from build123d import *

# Parameters (mm, degrees)
F0_W      = 70
F0_H      = 40
F1_DEPTH  = 40
F3_DEPTH  = 70
F4_DEPTH  = 140
F6_DEPTH  = 40
F8_DEPTH  = 40
F9_DEPTH  = 80
F11_DEPTH = 10


with BuildPart() as f1:
    # F0 (on Front) → F1 (new body)
    with BuildSketch(Plane.XZ):
        with Locations((35, 20)):
            Rectangle(F0_W, F0_H)
    extrude(amount=F1_DEPTH)

    # F2 (on face) → F3 (join)
    with BuildSketch(Plane.YZ.offset(70)):
        Polygon((-20, 40), (-40, 40), (-40, 20), align=None)
    extrude(amount=F3_DEPTH)

    # F3_face (on face) → F4 (cut)
    with BuildSketch(Plane(origin=(140, -33.333333, 33.333333), x_dir=(0, 1, 0), z_dir=(1, 0, 0))):
        Polygon((13.333333, 6.666667), (-6.666667, 6.666667), (-6.666667, -13.333333), align=None)
    extrude(amount=-F4_DEPTH, mode=Mode.SUBTRACT)

    # F5 (on face) → F6 (cut)
    with BuildSketch(Plane(origin=(0, 0, 0), x_dir=(-1, 0, 0), z_dir=(0, 1, 0))):
        Polygon((-70, 40), (-70, 20), (-30, 40), align=None)
    extrude(amount=-F6_DEPTH, mode=Mode.SUBTRACT)

    # F7 (on face) → F8 (join)
    with BuildSketch(Plane(origin=(0, 0, 0), x_dir=(1, 0, 0), z_dir=(0, 0, -1))):
        Polygon((70, 20), (70, 40), (30, 40), align=None)
    extrude(amount=F8_DEPTH)

    # F8_face (on face) → F9 (cut)
    with BuildSketch(Plane(origin=(56.666667, -33.333333, -40), x_dir=(1, 0, 0), z_dir=(0, 0, -1))):
        Polygon((13.333333, -13.333333), (13.333333, 6.666667), (-26.666667, 6.666667), align=None)
    extrude(amount=-F9_DEPTH, mode=Mode.SUBTRACT)

    # F10 (on face) → F11 (join)
    with BuildSketch(Plane(origin=(0, -30, 30), x_dir=(1, 0, 0), z_dir=(0, -0.707107, 0.707107))):
        Polygon((50, 0), (30, 14.142136), (30, -14.142136), align=None)
    extrude(amount=-F11_DEPTH)


solid = f1.part
Geometry check sheet. Reference: the model listing, model coordinates, mm. Give positions to 0.01 mm unless a question says otherwise; leave off trailing zeros. Loops run counter-clockwise (first coordinate to the right, second up) from the corner with the lowest first, then second, coordinate; pieces in that order, holes last. Notation, with made-up numbers: (-23.5, 64.25) -> (0.5, 64.25) arc R22 cw to (0.5, 100.25) -> close; hole circle Ø9 at (-13.75, 45.25). An arc over 180 degrees is marked (long way). Answer in a Markdown table with one row per item. Add a question column.
1) Gauge pin test, flat ends, axial feed: P1, Ø4, axis at x = 22, z = 28, coming from the -Y side; P2, Ø1.5, axis at y = -19, z = 31.5, coming from the +X side. Record the tip position at first contact, or that the pin passes through.
2) Cross-section at C-C on x = 54.5. Record the boundary of the cut face in (y, z), and give its area (3 significant figures).
3) Cross-section at B-B on x = 35. Record the boundary of the cut face in (y, z), and give its area (3 significant figures).
4) Material ranges on probe 1 along Y at (x, z) = (49.5, 8.5); probe 2 along Y at (x, z) = (7.5, 25); probe 3 along Z at (x, y) = (42.5, -31.5), recorded low to high. Write a range as from..to.
5) Cross-section at A-A on z = 11. Record the boundary of the cut face in (x, y).
Outcome:
| question | item | result |
|---|---|---|
| 1 | P1 | stops at y = -34 |
| 1 | P2 | stops at x = 48.5 |
| 2 | outline | (-27.75, 0) -> (0, 0) -> (0, 27.75) -> (-27.75, 27.75) -> close |
| 2 | area | 770 mm^2 |
| 3 | outline | (-37.5, 0) -> (0, 0) -> (0, 37.5) -> (-22.5, 37.5) -> (-37.5, 22.5) -> close |
| 3 | area | 1,290 mm^2 |
| 4 | probe 1 | y = -30.25..0 |
| 4 | probe 2 | y = -35..0 |
| 4 | probe 3 | z = 0..28.5 |
| 5 | outline | (0, -40) -> (30, -40) -> (70, -20) -> (70, 0) -> (0, 0) -> close |
